```python
from build123d import *

# Parameters (mm, degrees)
F0_W      = 150.1006782055
F0_H      = 110.9899356961
F1_DEPTH  = 92.4
F2_W      = 150.1006782055
F2_H      = 19.9922849774
F3_DEPTH  = 28.7
F4_W      = 150.1006782055
F4_H      = 6.7310594022
F5_DEPTH  = 18.5
F6_W      = 141.5597423911
F6_H      = 12.2390463948
F7_DEPTH  = 9.7
F8_W      = 132.9917162657
F8_H      = 56.4299700782
F9_DEPTH  = 2.5
F10_R     = 6.077615329
F10_R_2   = 6.1309658988
F10_R_3   = 6.1687846494
F10_R_4   = 6.0083305598
F11_DEPTH = 5
F12_R     = 12.3227416523
F12_R_2   = 11.0367187647
F12_R_3   = 12.1926494199
F12_R_4   = 11.2992603937
F12_R_5   = 12.1037249709
F12_R_6   = 11.2032484042
F12_R_7   = 12.0227070788
F12_R_8   = 10.9242891597
F12_R_9   = 8.3209245573
F12_R_10  = 7.3212092862
F12_R_11  = 8.1775044527
F12_R_12  = 7.3141816182
F12_R_13  = 8.0443237324
F12_R_14  = 6.796531977
F12_R_15  = 7.6510346435
F12_R_16  = 6.7661892343
F13_DEPTH = 1


with BuildPart() as f1:
    # F0 (on Front) → F1 (new body)
    with BuildSketch(Plane.XZ):
        Rectangle(F0_W, F0_H)
    extrude(amount=F1_DEPTH)

    # F2 (on face) → F3 (join)
    with BuildSketch(Plane.XY.offset(55.4949678481)):
        with Locations((0, -82.4038575113)):
            Rectangle(F2_W, F2_H)
    extrude(amount=F3_DEPTH)

    # F4 (on face) → F5 (join)
    with BuildSketch(Plane(origin=(0, 0, 0), x_dir=(-1, 0, 0), z_dir=(0, 1, 0))):
        with Locations((0, 26.1929742992)):
            Rectangle(F4_W, F4_H)
    extrude(amount=F5_DEPTH)

    # F6 (on face) → F7 (cut)
    with BuildSketch(Plane.XY.offset(29.5585040003)):
        with Locations((3.7253e-06, 6.1195231974)):
            Rectangle(F6_W, F6_H)
    extrude(amount=-F7_DEPTH, mode=Mode.SUBTRACT)

    # F8 (on face) → F9 (cut)
    with BuildSketch(Plane(origin=(0, 0, 0), x_dir=(-1, 0, 0), z_dir=(0, 1, 0))):
        with Locations((0.6100535393, -13.5516175069)):
            Rectangle(F8_W, F8_H)
    extrude(amount=-F9_DEPTH, mode=Mode.SUBTRACT)

    # F10 (on face) → F11 (join)
    with BuildSketch(Plane(origin=(0, 0, 0), x_dir=(-1, 0, 0), z_dir=(0, 1, 0))):
        with Locations((-24.7071757913, 41.8107584119)):
            Circle(F10_R)
        with Locations((-59.7852654755, 41.8107584119)):
            Circle(F10_R_2)
        with Locations((24.4021452963, 41.8107584119)):
            Circle(F10_R_3)
        with Locations((57.0400170982, 41.8107584119)):
            Circle(F10_R_4)
    extrude(amount=F11_DEPTH)

    # F12 (on face) → F13 (join)
    with BuildSketch(Plane.XY.offset(55.4949678481)):
        with Locations((45.8669885993, -21.8506734818)):
            Circle(F12_R)
        with Locations((45.8669885993, -21.8506734818)):
            Circle(F12_R_2, mode=Mode.SUBTRACT)
        with Locations((-46.1877398193, -54.5669868588)):
            Circle(F12_R_3)
        with Locations((-46.1877398193, -54.5669868588)):
            Circle(F12_R_4, mode=Mode.SUBTRACT)
        with Locations((46.187736094, -54.5669868588)):
            Circle(F12_R_5)
        with Locations((46.187736094, -54.5669868588)):
            Circle(F12_R_6, mode=Mode.SUBTRACT)
        with Locations((-46.1877398193, -21.8506734818)):
            Circle(F12_R_7)
        with Locations((-46.1877398193, -21.8506734818)):
            Circle(F12_R_8, mode=Mode.SUBTRACT)
        with Locations((-46.1877398193, -54.5669868588)):
            Circle(F12_R_9)
        with Locations((-46.1877398193, -54.5669868588)):
            Circle(F12_R_10, mode=Mode.SUBTRACT)
        with Locations((-46.1877398193, -21.8506734818)):
            Circle(F12_R_11)
        with Locations((-46.1877398193, -21.8506734818)):
            Circle(F12_R_12, mode=Mode.SUBTRACT)
        with Locations((45.8669885993, -21.8506734818)):
            Circle(F12_R_13)
        with Locations((45.8669885993, -21.8506734818)):
            Circle(F12_R_14, mode=Mode.SUBTRACT)
        with Locations((46.187736094, -54.5669868588)):
            Circle(F12_R_15)
        with Locations((46.187736094, -54.5669868588)):
            Circle(F12_R_16, mode=Mode.SUBTRACT)
    extrude(amount=F13_DEPTH)


solid = f1.part
```
Work out the finished part from the listing and answer in its coordinate system (mm). A direction names the side the tool comes from. Give positions to 0.01 mm unless a question says otherwise; leave off trailing zeros. Write each loop counter-clockwise with the first axis right and the second up, starting at its lowest first coordinate (ties: lowest second). Pieces come first, ordered by that corner, then holes.
(1) The part is cut by section B-B on y = 8. Write down the section's boundary in (x, z), plus the area to 3 significant figures.
Final values:
outline: (-75.05, 22.83) - (-70.78, 22.83) - (-70.78, 29.56) - (-75.05, 29.56) - close; (70.78, 22.83) - (75.05, 22.83) - (75.05, 29.56) - (70.78, 29.56) - close
area: 57.5 mm2
(2) The part is cut by section C-C on z = -30. Write down the section's boundary in (x, y), plus the area to 3 significant figures.
Final values:
outline: (-75.05, -92.4) - (75.05, -92.4) - (75.05, 0) - (65.89, 0) - (65.89, -2.5) - (-67.11, -2.5) - (-67.11, 0) - (-75.05, 0) - close
area: 13,500 mm2
(3) The part is cut by section D-D on y = -39. Write down the section's boundary in (x, z).
Final values:
outline: (-75.05, -55.49) - (75.05, -55.49) - (75.05, 55.49) - (-75.05, 55.49) - close
(4) Straight lines are drawn through the part: line 1 (Y direction, x = -24, z = 25.5); line 2 (X direction, y = 1.5, z = 46); line 3 (Y direction, x = -49, z = 51). For each, find the intervals that lie inside material, in ascending order.
Final values:
line 1: y = -92.4 to 0, 12.24 to 18.5
line 2: x = -61.35 to -52.73, -28.93 to -19.87, 20.3 to 29.11, 55.31 to 64.26
line 3: y = -92.4 to 0
(5) Flat-ended cylindrical pins translate along their axes: pin 1 Ø10 at (x, y) = (32, -17.5) entering from +Z; pin 2 Ø10 at (x, y) = (25.5, -61) entering from +Z. Find the tip coordinate at first contact, or state that the pin passes through.
Final values:
pin 1: stops at z = 56.49
pin 2: stops at z = 55.49
(6) The mould has two halves that part along Y. Classify faces 5 (the flat face through (-41, -60, 56.495)), 6 (the flat face through (60, 5, 42)), 7 (the cylindrical face through (-39.63, -44.29, 55.99)): pulls with the +Y half, pulls with the -Y half, needs draft (parallel to the pull), parting line crosses it, or undercut.
Final values:
face 5: needs draft
face 6: pulls with the +Y half
face 7: undercut
(7) Which of the six approach directions +Z, -Z, +X, -X, +Y, -Y give full straight-line access (tool end or side, diameter ignored) to faces 1 (the cylindrical face through (-23.599, 2.465, 47.927)), 2 (the flat face through (-35, -58, 56.495)), 3 (the cylindrical face through (50.301, -48.116, 55.988)), 4 (the flat face through (0, 15, 22.827))?
Final values:
face 1: +Y
face 2: +Z, +X, -X, +Y
face 3: +Z
face 4: -Z, +X, -X, +Y
(8) The part is cut by section A-A on x = -3. Write down the section's boundary in (y, z), plus the area to 3 significant figures.
Final values:
outline: (-92.4, -55.49) - (0, -55.49) - (0, -41.77) - (-2.5, -41.77) - (-2.5, 14.66) - (0, 14.66) - (0, 55.49) - (-72.41, 55.49) - (-72.41, 84.19) - (-92.4, 84.19) - close; (12.24, 22.83) - (18.5, 22.83) - (18.5, 29.56) - (12.24, 29.56) - close
area: 10,700 mm2
